Can you work these out from the model? Positions are in its coordinate system, mm. A direction names the side the tool comes from. Coordinates: 2 decimals unless noted, no trailing zeros. Order: outer loops, then holes, each group sorted by start corner. A loop starts at its lowest first (then second) coordinate and runs counter-clockwise, first axis right, second up. Notation, with made-up numbers: M 69,49.25 L 90,49.25 A13 ccw 90,59.25 Z; hole C 16,39 d8. An arc over 180 degrees is marked long. Answer as CSV lines item,"result". Start each with the question number.
1. If we mould it in two halves opening along X, with no side actions, what happens to faces 4 (the face through (-9.5, 0.07, 1.48)), 5 (the face through (-5, 15, 1)), 6 (the face through (9, 13, 1))? For each: released by +X, released by -X, zero draft, split by the parting line, or undercut.
2. If we section it at C-C (y = 0): List the corners of the cut face in (x, z) for me.
3. If we section it at B-B (z = 1.65): List the corners of the cut face in (x, y) for me.
4. On a 3-axis mill with a long thin cutter (end or side, diameter ignored), from which of +Z, -Z, +X, -X, +Y, -Y can I reach the whole of each face in a straight line? I mean faces 1 (the face through (6.5, 0.07, 1.48)), 2 (the face through (5, 14, 1)), 3 (the face through (-9, 13, 1)). Say none if no direction works.
5. Will these pins go through, and if not, where does the flat tip stop? pin 1 (1.5 mm diameter, centred on y = 14.5, z = 1, fed in from +X); pin 2 (6 mm diameter, centred on x = 0, y = 0, fed in from -Z); pin 3 (1.5 mm diameter, centred on y = 14.5, z = 1.5, fed in from -X).
6. If we section it at A-A (x = 0): List the corners of the cut face in (y, z) for me.
7. I need wall thicknesses on line 1 along Y through (x, z) = (8, 2); line 2 along Y through (x, z) = (0, 2.1); line 3 along Y through (x, z) = (11.25, 2.4). Which ranges of each line are inside material? Lowest first, please. Write a range as from..to.
8. If we section it at D-D (y = 4): List the corners of the cut face in (x, z) for me, plus the area to 3 significant figures.
```python
from build123d import *

# Parameters (mm, degrees)
SKETCH1_R           = 5.2
SKETCH1_R_2         = 1.5
BOSS_EXTRUDE1_DEPTH = 3


with BuildPart() as part:
    # Sketch1 → Boss-Extrude1 (new body)
    with BuildSketch(Plane.XY):
        Polygon((-12.5, 13), (-12.5, -12), (12.5, -12), (12.5, 13), (5, 13), (5, 16), (-5, 16), (-5, 13), align=None)
        Circle(SKETCH1_R, mode=Mode.SUBTRACT)
        with Locations((-8, 0)):
            Circle(SKETCH1_R_2, mode=Mode.SUBTRACT)
        with Locations((8, 0)):
            Circle(SKETCH1_R_2, mode=Mode.SUBTRACT)
    extrude(amount=BOSS_EXTRUDE1_DEPTH)


solid = part.part
```
Solved:
1,face 4,"undercut"
1,face 5,"released by -X"
1,face 6,"zero draft"
2,outline,"M -12.5,0 L -9.5,0 L -9.5,3 L -12.5,3 Z; M -6.5,0 L -5.2,0 L -5.2,3 L -6.5,3 Z; M 5.2,0 L 6.5,0 L 6.5,3 L 5.2,3 Z; M 9.5,0 L 12.5,0 L 12.5,3 L 9.5,3 Z"
3,outline,"M -12.5,-12 L 12.5,-12 L 12.5,13 L 5,13 L 5,16 L -5,16 L -5,13 L -12.5,13 Z; hole C -8,0 d3; hole C 0,0 d10.4; hole C 8,0 d3"
4,face 1,"+Z, -Z"
4,face 2,"+Z, -Z, +X, +Y"
4,face 3,"+Z, -Z, -X, +Y"
5,pin 1,"x = 5"
5,pin 2,"through"
5,pin 3,"x = -5"
6,outline,"M -12,0 L -5.2,0 L -5.2,3 L -12,3 Z; M 5.2,0 L 16,0 L 16,3 L 5.2,3 Z"
7,line 1,"-12..-1.5, 1.5..13"
7,line 2,"-12..-5.2, 5.2..16"
7,line 3,"-12..13"
8,outline,"M -12.5,0 L -3.32,0 L -3.32,3 L -12.5,3 Z; M 3.32,0 L 12.5,0 L 12.5,3 L 3.32,3 Z"
8,area,"55.1 mm²"
